```python
from build123d import *

# Parameters (mm, degrees)
SALIENTE_EXTRUIR1_DEPTH = 11
CROQUIS2_R              = 2
SALIENTE_EXTRUIR3_DEPTH = 16
CROQUIS3_R              = 2.05
CORTAR_EXTRUIR1_DEPTH   = 2
CROQUIS4_R              = 3.5
CORTAR_EXTRUIR2_DEPTH   = 4
CROQUIS5_W              = 4
CROQUIS5_H              = 7.2
CORTAR_EXTRUIR3_DEPTH   = 47.411205543
CROQUIS6_R              = 3
CORTAR_EXTRUIR4_DEPTH   = 47.411205543
CROQUIS7_R              = 6
CORTAR_EXTRUIR5_DEPTH   = 3


with BuildPart() as part:
    # Croquis1 → Saliente-Extruir1 (new body)
    with BuildSketch(Plane.XY):
        Polygon((17.320508076, 0), (8.660254038, 15), (-8.660254038, 15), (-17.320508076, 0), (-8.660254038, -15), (8.660254038, -15), align=None)
        Polygon((12.701705922, 0), (6.350852961, 11), (-6.350852961, 11), (-12.701705922, 0), (-6.350852961, -11), (6.350852961, -11), align=None, mode=Mode.SUBTRACT)
    extrude(amount=SALIENTE_EXTRUIR1_DEPTH)

    # Croquis2 → Saliente-Extruir3 (add)
    with BuildSketch(Plane.XY.offset(11)):
        Polygon((-8.660254038, 15), (-17.320508076, 0), (-8.660254038, -15), (8.660254038, -15), (17.320508076, 0), (8.660254038, 15), align=None)
        Circle(CROQUIS2_R, mode=Mode.SUBTRACT)
    extrude(amount=SALIENTE_EXTRUIR3_DEPTH)

    # Croquis3 → Cortar-Extruir1 (cut)
    with BuildSketch(Plane.XY.offset(27)):
        Circle(CROQUIS3_R)
    extrude(amount=-CORTAR_EXTRUIR1_DEPTH, mode=Mode.SUBTRACT)

    # Croquis4 → Cortar-Extruir2 (cut)
    with BuildSketch(Plane(origin=(0, 0, 11), x_dir=(-1, 0, 0), z_dir=(0, 0, -1))):
        Circle(CROQUIS4_R)
    extrude(amount=-CORTAR_EXTRUIR2_DEPTH, mode=Mode.SUBTRACT)

    # Croquis5 → Cortar-Extruir3 (cut, through all)
    with BuildSketch(Plane(origin=(-12.990381057, 7.5, 0), x_dir=(0, 0, 1), z_dir=(-0.8660254037844386, 0.5, 0))):
        with Locations((20, 0)):
            Rectangle(CROQUIS5_W, CROQUIS5_H)
    extrude(amount=-CORTAR_EXTRUIR3_DEPTH, mode=Mode.SUBTRACT)

    # Croquis6 → Cortar-Extruir4 (cut, through all)
    with BuildSketch(Plane(origin=(-12.990381057, 7.5, 0), x_dir=(0, 0, 1), z_dir=(-0.8660254037844386, 0.5, 0))):
        with Locations(Location((4.3, 0, 0), (0, 0, 270))):
            Circle(CROQUIS6_R)
    extrude(amount=-CORTAR_EXTRUIR4_DEPTH, mode=Mode.SUBTRACT)

    # Croquis7 → Cortar-Extruir5 (cut)
    with BuildSketch(Plane.XY.offset(27)):
        Polygon((-8.660254038, 15), (-17.320508076, 0), (-8.660254038, -15), (8.660254038, -15), (17.320508076, 0), (8.660254038, 15), align=None)
        Circle(CROQUIS7_R, mode=Mode.SUBTRACT)
    extrude(amount=-CORTAR_EXTRUIR5_DEPTH, mode=Mode.SUBTRACT)


solid = part.part
```
Source: CAD feature listing. Evaluate the final solid. Frame: model axes, mm. A direction names the side the tool comes from. Give positions to 0.01 mm unless a question says otherwise; leave off trailing zeros. Order: outer loops, then holes, each group sorted by start corner. A loop starts at its lowest first (then second) coordinate and runs counter-clockwise, first axis right, second up. Notation, with made-up numbers: (46.5, 59) -> (96.5, 59) arc R34 ccw to (96.5, 98) -> close; hole circle Ø3 at (-23, 72.5). An arc over 180 degrees is marked (long way). Use a Markdown table: item, result.
Q1. Section D-D (x = -7.5). Return the cut outline in (y, z).
A:
| item | result |
|---|---|
| outline | (-15, 0) -> (-9.01, 0) -> (-9.01, 11) -> (9.01, 11) -> (9.01, 0) -> (15, 0) -> (15, 24) -> (-15, 24) -> close; hole (0.17, 18) -> (8.49, 18) -> (8.49, 22) -> (0.17, 22) -> close |
Q2. First-contact query: P1, Ø10.5, axis at x = -1.5, y = 2.5, coming from the -Z side; P2, Ø3.5, axis at x = 0, y = 0, coming from the -Z side; P3, Ø1.5, axis at y = -4, z = 12, coming from the -X side; P4, Ø5, axis at y = 10.5, z = 21.5, coming from the +X side. Flat tips, straight axial feed; report the tip coordinate or a pass-through.
A:
| item | result |
|---|---|
| P1 | z = 11 |
| P2 | through |
| P3 | x = -15.44 |
| P4 | x = 12.7 |
Q3. Material intervals for line 1 (Z direction, x = 5.5, y = -2.5); line 2 (X direction, y = 0, z = 15.8); line 3 (Y direction, x = 1, z = 3.25), sorted ascending. Write a range as [from, to].
A:
| item | result |
|---|---|
| line 1 | [11, 18], [22, 24] |
| line 2 | [-17.32, -2], [2, 17.32] |
| line 3 | [-15, -11], [11, 15] |
Q4. Section A-A (z = 23). Return the cut outline in (x, y), and give its area (3 significant figures).
A:
| item | result |
|---|---|
| outline | (-17.32, 0) -> (-8.66, -15) -> (8.66, -15) -> (17.32, 0) -> (8.66, 15) -> (-8.66, 15) -> close; hole circle Ø4 at (0, 0) |
| area | 767 mm^2 |
Q5. Pull-direction query (Y, two-part tool) for faces 1 (the face through (0, 15, 12)), 2 (the face through (-13.05, -7.4, 11.83)), 3 (the face through (0, -2, 23)); classes: +Y half, -Y half, draft (parallel to the pull), parting line (faces both ways), or undercut.
A:
| item | result |
|---|---|
| face 1 | +Y half |
| face 2 | -Y half |
| face 3 | undercut |
Q6. Access query for faces 4 (the face through (-1, -2, 18)), 5 (the face through (7, 0, 24)), 6 (the face through (-2, -2, 15)). Directions: +Z, -Z, +X, -X, +Y, -Y. A direction counts if a zero-diameter tool reaches every point of the face in a straight line with its end or side. Return the directions, or none.
A:
| item | result |
|---|---|
| face 4 | none |
| face 5 | +Z |
| face 6 | -Z |
